Source: CAD feature listing. Evaluate the final solid. Frame: model axes, mm. A direction names the side the tool comes from. Coordinates: 2 decimals unless noted, no trailing zeros. Write each loop counter-clockwise with the first axis right and the second up, starting at its lowest first coordinate (ties: lowest second). Pieces come first, ordered by that corner, then holes. Notation, with made-up numbers: (44.25, -16.75) -> (49.25, -16.75) arc R16 cw to (49.25, 13.25) -> close; hole circle Ø2 at (-37.75, 26.5). An arc over 180 degrees is marked (long way). One line per item, written item: value. Start each with the question number.
1. Section query D-D, the plane y = 8. State how many separate pieces and enclosed holes the cut face has, and give its area (3 significant figures).
2. Section query A-A, the plane x = 0. Output: boundary loops of the cut face in (y, z) (3 decimals), and give its area (3 significant figures).
3. Line query: line 1 (X direction, y = 0.75, z = 8); line 2 (X direction, y = 5.5, z = -21.5); line 3 (X direction, y = 8.5, z = 23.5). Output: solid intervals per line, ascending.
4. Section query C-C, the plane z = 1. Output: boundary loops of the cut face in (x, y), and give its area (3 significant figures).
5. Access query for faces 1 (the cylindrical face through (-16.74, 4.93, -14.2)), 2 (the flat face through (4.5, 5.1, 27.8)), 3 (the flat face through (-21.64, 5.07, -17.69)), 4 (the flat face through (10, 4, 32)). Directions: +Z, -Z, +X, -X, +Y, -Y. A direction counts if a zero-diameter tool reaches every point of the face in a straight line with its end or side. Return the directions, or none.
6. Mould query, pull axis Z, two halves, no side actions, for faces 5 (the cylindrical face through (-32.615, 1.426, -10.503)), 6 (the flat face through (22.57, 3.82, 24.58)), 7 (the cylindrical face through (-29.812, 6.983, 8.885)), 8 (the flat face through (21.78, 5.07, -17.77)). Classes: released by +Z, released by -Z, zero draft, split by the parting line, or undercut.
7. Section query B-B, the plane z = -31. Output: boundary loops of the cut face in (x, y), and give its area (3 significant figures).
8. First-contact query: P1, Ø5, axis at y = 7, z = 27.5, coming from the -X side; P2, Ø4, axis at x = 8.25, z = 4.76, coming from the +Y side; P3, Ø1, axis at x = -26, y = 3.5, coming from the +Z side; P4, Ø5, axis at y = 4.5, z = -28.5, coming from the -X side. Flat tips, straight axial feed; report the tip coordinate or a pass-through.
from build123d import *

# Parameters (mm, degrees)
BOSS_EXTRUDE1_DEPTH      = 10
BOSS_EXTRUDE2_DEPTH      = 10
CUT_EXTRUDE1_REACH       = 47.069
FILLET1_R                = 5
F_4_0_MM_DOWEL_HOLES1_D  = 4
CIRPATTERN5_COUNT        = 6
FILLET1_OF_CIRPATTERN5_R = 5
FILLET2_R                = 2
SKETCH6_R                = 6.35
CUT_EXTRUDE2_DEPTH       = 51.71349811760731
M3_CLEARANCE_HOLE1_D     = 3.6
CIRPATTERN6_COUNT        = 3


with BuildPart() as part:
    # Sketch1 → Boss-Extrude1 (new body)
    with BuildSketch(Plane(origin=(0, 0, 0), x_dir=(1, 0, 0), z_dir=(0, 1, 0))):
        Polygon((-28.867513459481238, 4.38e-15), (-14.43375672974066, 25.000000000000057), (14.433756729740656, 25.000000000000057), (28.867513459481245, 6.61e-15), (14.433756729740656, -25.00000000000005), (-14.433756729740653, -25.00000000000005), align=None)
    extrude(amount=BOSS_EXTRUDE1_DEPTH)

    # Sketch2 → Boss-Extrude2 (add)
    with BuildSketch(Plane(origin=(21.650635094611008, 0, 12.49999999999995), x_dir=(0.49999999999999784, 0, -0.86602540378444), z_dir=(0.86602540378444, 0, 0.49999999999999784))):
        Polygon((-10.000000000000002, 10), (9.999999999999998, 10.000000000000004), (10, 3.67e-15), (-10, 0), align=None)
    boss_extrude2 = extrude(amount=BOSS_EXTRUDE2_DEPTH)

    # Sketch3 → Cut-Extrude1 (cut, up to next)
    with BuildSketch(Plane(origin=(0, 10, 0), x_dir=(1, 0, 0), z_dir=(0, 1, 0)), mode=Mode.PRIVATE) as cut_extrude1_sk1:
        Polygon((28.060889132455394, -21.397114317029995), (32.56088913245539, -13.602885682970053), (20.436533479473244, -6.602885682970054), (15.936533479473251, -14.39711431702999), align=None)
    cut_extrude1_tool1 = extrude(cut_extrude1_sk1.sketch, amount=-CUT_EXTRUDE1_REACH, mode=Mode.PRIVATE) & part.part
    cut_extrude1 = cut_extrude1_tool1.solids().sort_by_distance((24.248711, 10, 14))[0]
    add(cut_extrude1, mode=Mode.SUBTRACT)

    # Fillet1
    fillet1_edges = [part.edges().sort_by_distance(p)[0] for p in [
        (26.6858891324554, 5.1e-16, 23.778684177437157),
        (26.6858891324554, 10, 23.778684177437157),
        (33.935889132455365, 3.17e-15, 11.22131582256278),
        (33.935889132455365, 10.000000000000004, 11.22131582256278),
    ]]
    fillet(fillet1_edges, radius=FILLET1_R - 0.0001)  # a hair under: the kernel refuses the full size

    # Ø4.0 mm Dowel Holes1 (through all)
    with Locations(Plane(origin=(-4.999999999999981, -4.74e-15, 8.660254037844405), x_dir=(0.8660254037844399, 0, 0.4999999999999979), z_dir=(-0.49999999999999784, 0, 0.8660254037844398))):
        with Locations((30, 5)):
            f_4_0_mm_dowel_holes1 = Hole(F_4_0_MM_DOWEL_HOLES1_D / 2)

    # CirPattern5: Boss-Extrude2, Cut-Extrude1, Ø4.0 mm Dowel Holes1 ×6 about axis
    cirpattern5_axis = Axis((-8.6e-16, 0, -9.3e-16), (0, 1, 0))
    add([boss_extrude2.rotate(cirpattern5_axis, i * 360 / CIRPATTERN5_COUNT) for i in range(1, CIRPATTERN5_COUNT)])
    add([cut_extrude1.rotate(cirpattern5_axis, i * 360 / CIRPATTERN5_COUNT) for i in range(1, CIRPATTERN5_COUNT)], mode=Mode.SUBTRACT)
    add([f_4_0_mm_dowel_holes1.rotate(cirpattern5_axis, i * 360 / CIRPATTERN5_COUNT) for i in range(1, CIRPATTERN5_COUNT)], mode=Mode.SUBTRACT)

    # Fillet1 of CirPattern5
    fillet1_of_cirpattern5_edges = [part.edges().sort_by_distance(p)[0] for p in [
        (33.93588913245536, 5.1e-16, -11.221315822562872),
        (33.93588913245536, 10, -11.221315822562872),
        (26.685889132455333, 3.17e-15, -23.77868417743721),
        (26.68588913245533, 10.000000000000004, -23.778684177437214),
        (7.24999999999996, 5.1e-16, -35.00000000000003),
        (7.249999999999962, 10, -35.00000000000003),
        (-7.250000000000035, 3.17e-15, -35),
        (-7.250000000000035, 10.000000000000004, -35),
        (-26.6858891324554, 5.1e-16, -23.778684177437164),
        (-26.6858891324554, 10, -23.778684177437164),
        (-33.935889132455365, 3.17e-15, -11.221315822562786),
        (-33.935889132455365, 10.000000000000004, -11.221315822562786),
        (-33.93588913245536, 5.1e-16, 11.221315822562858),
        (-33.935889132455365, 10, 11.221315822562856),
        (-26.685889132455337, 3.17e-15, 23.7786841774372),
        (-26.685889132455337, 10.000000000000004, 23.7786841774372),
        (-7.249999999999951, 5.1e-16, 35.000000000000036),
        (-7.249999999999951, 10, 35.000000000000036),
        (7.250000000000045, 3.17e-15, 34.99999999999999),
        (7.2500000000000435, 10.000000000000004, 34.99999999999999),
    ]]
    fillet(fillet1_of_cirpattern5_edges, radius=FILLET1_OF_CIRPATTERN5_R - 0.0001)  # a hair under: the kernel refuses the full size

    # Fillet2
    fillet2_edges = [part.edges().sort_by_distance(p)[0] for p in [
        (-10.00000000000006, 5.0000000000000036, -24.99999999999999),
        (-16.65063509461103, 5, -21.160254037844354),
        (-26.650635094610987, 5.0000000000000036, -3.839745962155554),
        (-26.65063509461097, 5, 3.839745962155675),
        (-16.650635094610934, 5.0000000000000036, 21.160254037844428),
        (-9.999999999999936, 5, 25.000000000000043),
        (10.000000000000064, 5.0000000000000036, 24.999999999999986),
        (20.436533479473248, 5, -6.602885682970051),
        (15.936533479473255, 5, -14.39711431702999),
        (4.499999999999998, 5, -21.000000000000046),
        (-4.499999999999988, 5, -21.00000000000005),
        (-15.936533479473251, 5, -14.397114317029994),
        (-20.436533479473244, 5, -6.602885682970059),
        (-20.43653347947325, 5, 6.602885682970041),
        (-15.93653347947326, 5, 14.397114317029978),
        (-4.499999999999992, 5, 21.000000000000043),
        (4.499999999999993, 5, 21.000000000000043),
        (16.65063509461103, 5, 21.16025403784435),
        (26.650635094610987, 5.0000000000000036, 3.8397459621555505),
        (15.936533479473251, 5, 14.39711431702999),
        (20.436533479473244, 5, 6.602885682970054),
        (26.65063509461097, 5, -3.8397459621556855),
        (16.650635094610927, 5.0000000000000036, -21.160254037844435),
        (9.999999999999943, 5, -25.00000000000004),
    ]]
    fillet(fillet2_edges, radius=FILLET2_R)

    # Sketch6 → Cut-Extrude2 (cut, through all)
    with BuildSketch(Plane(origin=(0, 10, 0), x_dir=(1, 0, 0), z_dir=(0, 1, 0))):
        with Locations(Location((0, 0, 0), (0, 0, 270))):
            Circle(SKETCH6_R)
    extrude(amount=-CUT_EXTRUDE2_DEPTH, mode=Mode.SUBTRACT)

    # M3 Clearance Hole1 (through all)
    with Locations(Plane(origin=(0, 10, 0), x_dir=(1, 0, 0), z_dir=(0, 1, 0))):
        with Locations((0, 9.525)):
            m3_clearance_hole1 = Hole(M3_CLEARANCE_HOLE1_D / 2)

    # CirPattern6: M3 Clearance Hole1 ×3 about axis
    cirpattern6_axis = Axis((-3.1e-16, 0, 4.7e-16), (0, 1, 0))
    for i in range(1, CIRPATTERN6_COUNT):
        add(m3_clearance_hole1.rotate(cirpattern6_axis, i * 360 / CIRPATTERN6_COUNT), mode=Mode.SUBTRACT)


solid = part.part
Computed values:
1. separate pieces: 1
1. enclosed holes: 4
1. area: 2,410 mm²
2. outline: (0, -21) -> (10, -21) -> (10, -11.325) -> (0, -11.325) -> close; (0, -7.725) -> (10, -7.725) -> (10, -6.35) -> (0, -6.35) -> close; (0, 6.35) -> (10, 6.35) -> (10, 21) -> (0, 21) -> close
2. area: 257 mm²
3. line 1: x = -33.06 to -22.86, -19.68 to 19.68, 22.86 to 33.06
3. line 2: x = -27.97 to -24.46, -19.99 to -3.82, 3.82 to 19.99, 24.46 to 27.97
3. line 3: x = -25.2 to -20.7, -15.3 to -4.5, 4.5 to 15.3, 20.7 to 25.2
4. outline: (-28.29, 0) -> (-6.27, 0) -> (-6.27, 10) -> (-28.29, 10) -> close; (6.27, 0) -> (28.29, 0) -> (28.29, 10) -> (6.27, 10) -> close
4. area: 440 mm²
5. face 1: +Y, -Y
5. face 2: +Z, +Y, -Y
5. face 3: -X, +Y, -Y
5. face 4: +Z, +X, +Y, -Y
6. face 5: released by -Z
6. face 6: released by +Z
6. face 7: undercut
6. face 8: undercut
7. outline: (-10, 0.1) -> (-4.5, 0.1) -> (-4.5, 3.27) -> (-10, 3.27) -> close; (-10, 6.73) -> (-4.5, 6.73) -> (-4.5, 9.9) -> (-10, 9.9) -> close; (4.5, 0.1) -> (10, 0.1) -> (10, 3.27) -> (4.5, 3.27) -> close; (4.5, 6.73) -> (10, 6.73) -> (10, 9.9) -> (4.5, 9.9) -> close
7. area: 69.7 mm²
8. P1: stops at x = -25.74
8. P2: stops at y = 10
8. P3: stops at z = 25.42
8. P4: stops at x = -25.39
